Build history of the part. All positions in model axes, mm. Give positions to 0.01 mm unless a question says otherwise; leave off trailing zeros. Write each loop counter-clockwise with the first axis right and the second up, starting at its lowest first coordinate (ties: lowest second). Pieces come first, ordered by that corner, then holes. Notation, with made-up numbers: (62.5, 65.5) - (96.5, 65.5) arc R14 ccw to (96.5, 73.5) - close; hole circle Ø2 at (-11.5, -29.5). An arc over 180 degrees is marked (long way). Use one line per item in the form item = value. Start each with the question number.
from build123d import *

# Parameters (mm, degrees)
SURFACE_EXTRUDE4_START     = -1.778
SURFACE_EXTRUDE4_OUTLINE_R = 1.709503837
SURFACE_EXTRUDE4_DEPTH     = 14.986


# Read off the part's stored shape, not the designer's step: Surface-Extrude4
with BuildPart() as part:
    # Surface-Extrude4 outline → Surface-Extrude4 (new body)
    with BuildSketch(Plane.ZY.offset(-0.2921).offset(SURFACE_EXTRUDE4_START)):
        with Locations((37.259820513, -0.026967113)):
            Circle(SURFACE_EXTRUDE4_OUTLINE_R)
    extrude(amount=SURFACE_EXTRUDE4_DEPTH)


solid = part.part
(1) Two-plate mould, pull along X, no slides. Class faces 1 (the flat face through (2.07, 0, 37)), 2 (the flat face through (-12.916, 0, 37)), 3 (the cylindrical face through (-5.32, -0.68, 38.84)): +X half, -X half, draft (parallel to the pull), parting line (faces both ways), or undercut.
(2) Wall check: line 1 (Y direction, x = -4, z = 37.35); line 2 (Y direction, x = -1, z = 38.3); line 3 (Z direction, x = -1, y = -0.65). Give the ranges that are in metal, low to high. Write a range as from..to.
(3) Cut at A-A, the plane x = -5.5. Give the cut face in (y, z).
(4) Cut at C-C, the plane y = 1.15. Give the cut face in (x, z).
(5) Cut at B-B, the plane z = 38.5. Give the cut face in (x, y), then the cut area to 3 significant figures.
(6) Pin check, flat tips, straight feed: pin 1 Ø2 at (x, y) = (-8, 0.5) entering from +Z; pin 2 Ø1.5 at (x, y) = (-5.5, -1.5) entering from +Z. Stop position of each tip, or through.
Solution:
q1.face_1 = +X half
q1.face_2 = -X half
q1.face_3 = draft
q2.line_1 = -1.73..1.68
q2.line_2 = -1.38..1.33
q2.line_3 = 35.67..38.85
q3.outline = circle Ø3.42 at (-0.03, 37.26)
q4.outline = (-12.92, 36.02) - (2.07, 36.02) - (2.07, 38.5) - (-12.92, 38.5) - close
q5.outline = (-12.92, -1.2) - (2.07, -1.2) - (2.07, 1.15) - (-12.92, 1.15) - close
q5.area = 35.3 mm2
q6.pin_1 = 38.97
q6.pin_2 = 38.81
